Work out the finished part from the listing and answer in its coordinate system (mm). A direction names the side the tool comes from. Give positions to 0.01 mm unless a question says otherwise; leave off trailing zeros. Loops run counter-clockwise (first coordinate to the right, second up) from the corner with the lowest first, then second, coordinate; pieces in that order, holes last. Notation, with made-up numbers: (30, -10.75) - (53, -10.75) arc R12 ccw to (53, 8.25) - close; hole circle Ø10 at (-1, 49.5). An arc over 180 degrees is marked (long way). Use one line per item in the form item = value. Start each with the question number.
from build123d import *

# Parameters (mm, degrees)
EXTRUDE_1_DEPTH     = 16
SKETCH_2_R          = 77.5
CUT_EXTRUDE_1_DEPTH = 1
CUT_EXTRUDE_2_REACH = 344.025
SKETCH_3_R          = 9
CUT_EXTRUDE_3_REACH = 344.07
CHAMFER_1_SIZE      = 10


with BuildPart() as part:
    # 草图1 → 凸台-拉伸1 (new body)
    with BuildSketch(Plane.XY):
        with BuildLine():
            Line((-74.306819623, 35.843361414), (-187.020661681, -197.82353813))
            ThreePointArc((-187.020661681, -197.82353813), (-189.245682164, -204.172424177), (-190, -210.857487736))
            Line((-190, -210.857487736), (-190, -284))
            Line((-190, -284), (0, -284))
            Line((0, -284), (190, -284))
            Line((190, -284), (190, -210.857487736))
            ThreePointArc((190, -210.857487736), (189.245682164, -204.172424177), (187.020661681, -197.82353813))
            Line((187.020661681, -197.82353813), (74.306819623, 35.843361414))
            ThreePointArc((74.306819623, 35.843361414), (0, 82.5), (-74.306819623, 35.843361414))
        make_face()
    extrude(amount=EXTRUDE_1_DEPTH)

    # 草图2 → 切除-拉伸1 (cut)
    with BuildSketch(Plane.XY.offset(16)):
        Circle(SKETCH_2_R)
    extrude(amount=-CUT_EXTRUDE_1_DEPTH, mode=Mode.SUBTRACT)

    # 草图3 → 切除-拉伸2 (cut, up to next)
    with BuildSketch(Plane.XY.offset(15), mode=Mode.PRIVATE) as cut_extrude_2_sk1:
        with Locations((0, 62.5)):
            Circle(SKETCH_3_R)
    cut_extrude_2_tool1 = extrude(cut_extrude_2_sk1.sketch, amount=-CUT_EXTRUDE_2_REACH, mode=Mode.PRIVATE) & part.part
    # 草图3 → 切除-拉伸2 (cut, up to next)
    with BuildSketch(Plane.XY.offset(15), mode=Mode.PRIVATE) as cut_extrude_2_sk2:
        with Locations((31.25, 54.126587737)):
            Circle(SKETCH_3_R)
    cut_extrude_2_tool2 = extrude(cut_extrude_2_sk2.sketch, amount=-CUT_EXTRUDE_2_REACH, mode=Mode.PRIVATE) & part.part
    # 草图3 → 切除-拉伸2 (cut, up to next)
    with BuildSketch(Plane.XY.offset(15), mode=Mode.PRIVATE) as cut_extrude_2_sk3:
        with Locations((54.126587737, 31.25)):
            Circle(SKETCH_3_R)
    cut_extrude_2_tool3 = extrude(cut_extrude_2_sk3.sketch, amount=-CUT_EXTRUDE_2_REACH, mode=Mode.PRIVATE) & part.part
    # 草图3 → 切除-拉伸2 (cut, up to next)
    with BuildSketch(Plane.XY.offset(15), mode=Mode.PRIVATE) as cut_extrude_2_sk4:
        with Locations((62.5, 0)):
            Circle(SKETCH_3_R)
    cut_extrude_2_tool4 = extrude(cut_extrude_2_sk4.sketch, amount=-CUT_EXTRUDE_2_REACH, mode=Mode.PRIVATE) & part.part
    # 草图3 → 切除-拉伸2 (cut, up to next)
    with BuildSketch(Plane.XY.offset(15), mode=Mode.PRIVATE) as cut_extrude_2_sk5:
        with Locations((54.126587737, -31.25)):
            Circle(SKETCH_3_R)
    cut_extrude_2_tool5 = extrude(cut_extrude_2_sk5.sketch, amount=-CUT_EXTRUDE_2_REACH, mode=Mode.PRIVATE) & part.part
    # 草图3 → 切除-拉伸2 (cut, up to next)
    with BuildSketch(Plane.XY.offset(15), mode=Mode.PRIVATE) as cut_extrude_2_sk6:
        with Locations((31.25, -54.126587737)):
            Circle(SKETCH_3_R)
    cut_extrude_2_tool6 = extrude(cut_extrude_2_sk6.sketch, amount=-CUT_EXTRUDE_2_REACH, mode=Mode.PRIVATE) & part.part
    # 草图3 → 切除-拉伸2 (cut, up to next)
    with BuildSketch(Plane.XY.offset(15), mode=Mode.PRIVATE) as cut_extrude_2_sk7:
        with Locations((0, -62.5)):
            Circle(SKETCH_3_R)
    cut_extrude_2_tool7 = extrude(cut_extrude_2_sk7.sketch, amount=-CUT_EXTRUDE_2_REACH, mode=Mode.PRIVATE) & part.part
    # 草图3 → 切除-拉伸2 (cut, up to next)
    with BuildSketch(Plane.XY.offset(15), mode=Mode.PRIVATE) as cut_extrude_2_sk8:
        with Locations((-31.25, -54.126587737)):
            Circle(SKETCH_3_R)
    cut_extrude_2_tool8 = extrude(cut_extrude_2_sk8.sketch, amount=-CUT_EXTRUDE_2_REACH, mode=Mode.PRIVATE) & part.part
    # 草图3 → 切除-拉伸2 (cut, up to next)
    with BuildSketch(Plane.XY.offset(15), mode=Mode.PRIVATE) as cut_extrude_2_sk9:
        with Locations((-54.126587737, -31.25)):
            Circle(SKETCH_3_R)
    cut_extrude_2_tool9 = extrude(cut_extrude_2_sk9.sketch, amount=-CUT_EXTRUDE_2_REACH, mode=Mode.PRIVATE) & part.part
    # 草图3 → 切除-拉伸2 (cut, up to next)
    with BuildSketch(Plane.XY.offset(15), mode=Mode.PRIVATE) as cut_extrude_2_sk10:
        with Locations((-62.5, 0)):
            Circle(SKETCH_3_R)
    cut_extrude_2_tool10 = extrude(cut_extrude_2_sk10.sketch, amount=-CUT_EXTRUDE_2_REACH, mode=Mode.PRIVATE) & part.part
    # 草图3 → 切除-拉伸2 (cut, up to next)
    with BuildSketch(Plane.XY.offset(15), mode=Mode.PRIVATE) as cut_extrude_2_sk11:
        with Locations((-54.126587737, 31.25)):
            Circle(SKETCH_3_R)
    cut_extrude_2_tool11 = extrude(cut_extrude_2_sk11.sketch, amount=-CUT_EXTRUDE_2_REACH, mode=Mode.PRIVATE) & part.part
    # 草图3 → 切除-拉伸2 (cut, up to next)
    with BuildSketch(Plane.XY.offset(15), mode=Mode.PRIVATE) as cut_extrude_2_sk12:
        with Locations((-31.25, 54.126587737)):
            Circle(SKETCH_3_R)
    cut_extrude_2_tool12 = extrude(cut_extrude_2_sk12.sketch, amount=-CUT_EXTRUDE_2_REACH, mode=Mode.PRIVATE) & part.part
    add(cut_extrude_2_tool1.solids().sort_by_distance((0, 62.5, 15))[0], mode=Mode.SUBTRACT)
    add(cut_extrude_2_tool2.solids().sort_by_distance((31.25, 54.126588, 15))[0], mode=Mode.SUBTRACT)
    add(cut_extrude_2_tool3.solids().sort_by_distance((54.126588, 31.25, 15))[0], mode=Mode.SUBTRACT)
    add(cut_extrude_2_tool4.solids().sort_by_distance((62.5, 0, 15))[0], mode=Mode.SUBTRACT)
    add(cut_extrude_2_tool5.solids().sort_by_distance((54.126588, -31.25, 15))[0], mode=Mode.SUBTRACT)
    add(cut_extrude_2_tool6.solids().sort_by_distance((31.25, -54.126588, 15))[0], mode=Mode.SUBTRACT)
    add(cut_extrude_2_tool7.solids().sort_by_distance((0, -62.5, 15))[0], mode=Mode.SUBTRACT)
    add(cut_extrude_2_tool8.solids().sort_by_distance((-31.25, -54.126588, 15))[0], mode=Mode.SUBTRACT)
    add(cut_extrude_2_tool9.solids().sort_by_distance((-54.126588, -31.25, 15))[0], mode=Mode.SUBTRACT)
    add(cut_extrude_2_tool10.solids().sort_by_distance((-62.5, 0, 15))[0], mode=Mode.SUBTRACT)
    add(cut_extrude_2_tool11.solids().sort_by_distance((-54.126588, 31.25, 15))[0], mode=Mode.SUBTRACT)
    add(cut_extrude_2_tool12.solids().sort_by_distance((-31.25, 54.126588, 15))[0], mode=Mode.SUBTRACT)

    # 草图4 → 切除-拉伸3 (cut, up to next)
    with BuildSketch(Plane.XY.offset(16), mode=Mode.PRIVATE) as cut_extrude_3_sk1:
        with BuildLine():
            Line((-145, -209), (145, -209))
            ThreePointArc((145, -209), (170, -234), (145, -259))
            Line((145, -259), (-145, -259))
            ThreePointArc((-145, -259), (-170, -234), (-145, -209))
        make_face()
    cut_extrude_3_tool1 = extrude(cut_extrude_3_sk1.sketch, amount=-CUT_EXTRUDE_3_REACH, mode=Mode.PRIVATE) & part.part
    add(cut_extrude_3_tool1.solids().sort_by_distance((0, -234, 16))[0], mode=Mode.SUBTRACT)

    # 倒角1
    chamfer_1_edges = [part.edges().sort_by_distance(p)[0] for p in [
        (190, -284, 8),
        (-190, -284, 8),
    ]]
    chamfer(chamfer_1_edges, length=CHAMFER_1_SIZE)


solid = part.part
1) Find the intervals of material crossed by probe 1 along Y at (x, z) = (-31.25, 11); probe 2 along Y at (x, z) = (7.5, 11); probe 3 along X at (y, z) = (-54.5, 14.5), in increasing order.
2) Determine the mould class of faces 1 (the flat face through (185, -279, 8)), 2 (the flat face through (-190, -242, 8)), 3 (the cylindrical face through (-38.39, 48.65, 7.6)), 4 (the cylindrical face through (169.994, -233.45, 8.112)) for opening direction X: released by +X, released by -X, zero draft, split by the parting line, or undercut.
3) Flat-ended cylindrical pins translate along their axes: pin 1 Ø8 at (x, z) = (-47, 5.5) entering from +Y; pin 2 Ø20.5 at (x, y) = (0, -62.5) entering from -Z; pin 3 Ø16 at (x, y) = (-54.13, 31.25) entering from +Z; pin 4 Ø23.5 at (x, y) = (62.5, 0) entering from +Z. Find the tip coordinate at first contact, or state that the pin passes through.
4) A cutting plane is placed at C-C (x = 155.5). Give the vertices of the cut face in (y, z).
5) A cutting plane is placed at D-D (z = 8.25). State how many separate pieces and enclosed holes the cut face has, plus the area to 3 significant figures.
6) A cutting plane is placed at B-B (x = 0). Give the vertices of the cut face in (y, z).
7) A cutting plane is placed at A-A (y = -234). Give the vertices of the cut face in (x, z).
8) A tool of negligible diameter and unlimited length cuts with its end or side. For faces 5 (the cylindrical face through (-189.225, -204.08, 7.888)), 6 (the flat face through (-1, 1, 15)), 7 (the cylindrical face through (-169.994, -234.55, 8.112)), from which of +Z, -Z, +X, -X, +Y, -Y can it reach the whole face along a straight path? Write none if from no direction.
Answer sheet:
q1.probe_1 = -284 to -259, -209 to -63.13, -45.13 to 45.13, 63.13 to 76.35
q1.probe_2 = -284 to -259, -209 to -67.47, -57.53 to 57.53, 67.47 to 82.16
q1.probe_3 = -117.89 to -40.24, -22.26 to -4.12, 4.12 to 22.26, 40.24 to 117.89
q2.face_1 = released by +X
q2.face_2 = released by -X
q2.face_3 = undercut
q2.face_4 = undercut
q3.pin_1 = 70.41
q3.pin_2 = 0
q3.pin_3 = through
q3.pin_4 = 15
q4.outline = (-284, 0) - (-256.69, 0) - (-256.69, 16) - (-284, 16) - close; (-211.31, 0) - (-132.48, 0) - (-132.48, 16) - (-211.31, 16) - close
q5.separate_pieces = 1
q5.enclosed_holes = 13
q5.area = 79,100 mm²
q6.outline = (-284, 0) - (-259, 0) - (-259, 16) - (-284, 16) - close; (-209, 0) - (-71.5, 0) - (-71.5, 15) - (-77.5, 15) - (-77.5, 16) - (-209, 16) - close; (-53.5, 0) - (53.5, 0) - (53.5, 15) - (-53.5, 15) - close; (71.5, 0) - (82.5, 0) - (82.5, 16) - (77.5, 16) - (77.5, 15) - (71.5, 15) - close
q7.outline = (-190, 0) - (-170, 0) - (-170, 16) - (-190, 16) - close; (170, 0) - (190, 0) - (190, 16) - (170, 16) - close
q8.face_5 = +Z, -Z, -X, +Y
q8.face_6 = +Z
q8.face_7 = +Z, -Z
